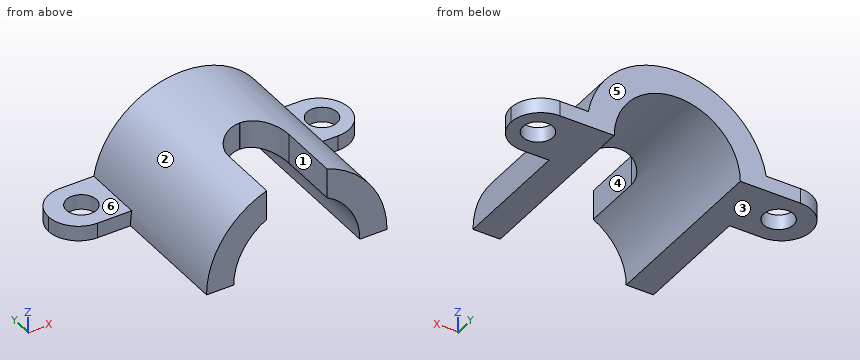
```python
from build123d import *

# Parameters (mm, degrees)
F1_W      = 30
F1_H      = 60
F2_ANGLE  = 180
F3_W      = 100
F3_H      = 20
F4_DEPTH  = 5
F5_R      = 9.99999
F6_R      = 5
F7_DEPTH  = 30.001
F8_W      = 20
F8_H      = 30
F9_DEPTH  = 30.001
F10_R     = 9.999
F11_R     = 20.9596675634
F12_DEPTH = 60.0010001


# Not quite as in the source:
# - a fillet or chamfer is up to 0.001 mm smaller than in the source, because OpenCascade refuses the exact size


with BuildPart() as f2:
    # F1 (on Top) → F2 (revolve)
    with BuildSketch(Plane.XY):
        with Locations((15, 30)):
            Rectangle(F1_W, F1_H)
    revolve(axis=Axis((0, 30, 0), (0, -1, 0)), revolution_arc=F2_ANGLE)

    # F3 (on Top) → F4 (join)
    with BuildSketch(Plane.XY):
        with Locations((-0.9596675634, 50)):
            Rectangle(F3_W, F3_H)
    extrude(amount=F4_DEPTH)

    # F5 (radius 10 in the source; OpenCascade refuses exactly that, so slightly less here)
    f5_edges = [f2.edges().sort_by_distance(p)[0] for p in [
        (-50.959668, 60, 2.5),
        (-50.959668, 40, 2.5),
        (49.040332, 40, 2.5),
        (49.040332, 60, 2.5),
    ]]
    fillet(f5_edges, radius=F5_R)

    # F6 (on Top) → F7 (cut, through all)
    with BuildSketch(Plane.XY):
        with Locations((40, 50)):
            Circle(F6_R)
        with Locations((-40, 50)):
            Circle(F6_R)
    extrude(amount=F7_DEPTH, mode=Mode.SUBTRACT)

    # F8 (on Top) → F9 (cut, through all)
    with BuildSketch(Plane.XY):
        with Locations((0, 15)):
            Rectangle(F8_W, F8_H)
    extrude(amount=F9_DEPTH, mode=Mode.SUBTRACT)

    # F10 (radius 10 in the source; OpenCascade refuses exactly that, so slightly less here)
    f10_edges = [f2.edges().sort_by_distance(p)[0] for p in [
        (-10, 30, 14.142136),
        (10, 30, 14.142136),
    ]]
    fillet(f10_edges, radius=F10_R)

    # F11 (on face) → F12 (cut, through all)
    with BuildSketch(Plane(origin=(0, 60, 0), x_dir=(-1, 0, 0), z_dir=(0, 1, 0))):
        Circle(F11_R)
    extrude(amount=-F12_DEPTH, mode=Mode.SUBTRACT)


solid = f2.part
```
Geometry: final body of the model. Coordinates: model frame, mm. Face numbers are marked on the shaded views. A direction names the side the tool comes from. Give positions to 0.01 mm unless a question says otherwise; leave off trailing zeros. Loops run counter-clockwise (first coordinate to the right, second up) from the corner with the lowest first, then second, coordinate; pieces in that order, holes last. Notation, with made-up numbers: (-34, 64) - (-1, 64) arc R14 cw to (-1, 68) - close; hole circle Ø9 at (47.5, 53). An arc over 180 degrees is marked (long way). Answer as CSV lines item,"result". Start each with the question number.
(1) Section query C-C (z = 9). Output: boundary loops of the cut face in (x, y), and give its area (3 significant figures).
(2) Reachability of the marked faces 4, 5 and 6 from +Z, -Z, +X, -X, +Y, -Y: full face, straight path, thin tool, end or side. Return the list, or none.
(3) Pin query (flat end, axial travel): P1, Ø2, axis at y = 42.5, z = 18.5, coming from the +X side; P2, Ø8, axis at y = 9, z = 23.5, coming from the -X side; P3, Ø6, axis at y = 8, z = 25, coming from the +X side. Return the tip coordinate at first contact, or that it passes through.
(4) Section query B-B (y = 54). Output: boundary loops of the cut face in (x, z), and give its area (3 significant figures).
(5) Mould query, pull axis X, two halves, no side actions, for the marked faces 1, 2 and 3. Classes: +X half, -X half, draft (parallel to the pull), parting line (faces both ways), or undercut.
(6) Section query A-A (z = 3.5). Give the number of separate pieces and of enclosed holes in the cut face, and give its area (3 significant figures).
(7) Ray query, line 1 along Y through (x, z) = (-40, 3.95); line 2 along X through (y, z) = (50, 3); line 3 along X through (y, z) = (50, 2.05). Return the intervals inside material, ascending. Write a range as [from, to].
(8) Section query D-D (x = 32.5). Output: boundary loops of the cut face in (y, z).
Worked answers:
1,outline,"(-28.62, 0) - (-18.93, 0) - (-18.93, 60) - (-28.62, 60) - close; (18.93, 0) - (28.62, 0) - (28.62, 60) - (18.93, 60) - close"
1,area,"1,160 mm^2"
2,face 4,"+Z, -Z, -Y"
2,face 5,"+Z, -Z, +X, -X, +Y"
2,face 6,"+Z, -X, +Y, -Y"
3,P1,"stops at x = 24.37"
3,P2,"stops at x = -22.8"
3,P3,"stops at x = 20.4"
4,outline,"(-50.12, 0) - (-43, 0) - (-43, 5) - (-50.12, 5) - close; (-37, 0) - (-20.96, 0) arc R20.96 cw to (20.96, 0) - (37, 0) - (37, 5) - (29.58, 5) arc R30 ccw to (-29.58, 5) - (-37, 5) - close; (43, 0) - (48.21, 0) - (48.21, 5) - (43, 5) - close"
4,area,"857 mm^2"
5,face 1,"undercut"
5,face 2,"parting line"
5,face 3,"draft"
6,separate pieces,"2"
6,enclosed holes,"2"
6,area,"1,660 mm^2"
7,line 1,"y = [40, 45], [55, 60]"
7,line 2,"x = [-50.96, -45], [-35, -20.74], [20.74, 35], [45, 49.04]"
7,line 3,"x = [-50.96, -45], [-35, -20.86], [20.86, 35], [45, 49.04]"
8,outline,"(40, 0) - (60, 0) - (60, 5) - (40, 5) - close"
